```python
from build123d import *

# Parameters (mm, degrees)
SKETCH1_R           = 19.36
BOSS_EXTRUDE1_DEPTH = 10
CUT_EXTRUDE1_REACH  = 12
CUT_EXTRUDE2_REACH  = 12
SKETCH3_R           = 9.21
SKETCH4_R           = 19.36
SKETCH4_R_2         = 9.21
BOSS_EXTRUDE2_DEPTH = 2
SKETCH5_R           = 19.522617412
SKETCH5_R_2         = 17.522617412
BOSS_EXTRUDE3_DEPTH = 12


with BuildPart() as part:
    # Sketch1 → Boss-Extrude1 (new body)
    with BuildSketch(Plane(origin=(0, 0, 0), x_dir=(1, 0, 0), z_dir=(0, 1, 0))):
        Circle(SKETCH1_R)
    extrude(amount=BOSS_EXTRUDE1_DEPTH)

    # Sketch2 → Cut-Extrude1 (cut, up to next)
    with BuildSketch(Plane.XZ, mode=Mode.PRIVATE) as cut_extrude1_sk1:
        with BuildLine():
            Line((13.175859246, 14.184721821), (10.029502225, 10.277095169))
            ThreePointArc((10.029502225, 10.277095169), (12.436124798, 7.18), (13.914976606, 3.54725613))
            Line((13.914976606, 3.54725613), (18.872259065, 4.318267913))
            ThreePointArc((18.872259065, 4.318267913), (16.766251817, 9.68), (13.175859246, 14.184721821))
        make_face()
    cut_extrude1_tool1 = extrude(cut_extrude1_sk1.sketch, amount=-CUT_EXTRUDE1_REACH, mode=Mode.PRIVATE) & part.part
    add(cut_extrude1_tool1.solids().sort_by_distance((14.534106, 0, 8.39127))[0], mode=Mode.SUBTRACT)
    # Sketch2 → Cut-Extrude1 (cut, up to next)
    with BuildSketch(Plane.XZ, mode=Mode.PRIVATE) as cut_extrude1_sk2:
        with BuildLine():
            ThreePointArc((-13.914976606, 3.54725613), (-12.436124798, 7.18), (-10.029502225, 10.277095169))
            Line((-10.029502225, 10.277095169), (-13.175859246, 14.184721821))
            ThreePointArc((-13.175859246, 14.184721821), (-16.766251817, 9.68), (-18.872259065, 4.318267913))
            Line((-18.872259065, 4.318267913), (-13.914976606, 3.54725613))
        make_face()
    cut_extrude1_tool2 = extrude(cut_extrude1_sk2.sketch, amount=-CUT_EXTRUDE1_REACH, mode=Mode.PRIVATE) & part.part
    add(cut_extrude1_tool2.solids().sort_by_distance((-14.534106, 0, 8.39127))[0], mode=Mode.SUBTRACT)
    # Sketch2 → Cut-Extrude1 (cut, up to next)
    with BuildSketch(Plane.XZ, mode=Mode.PRIVATE) as cut_extrude1_sk3:
        with BuildLine():
            Line((5.69639982, -18.502989734), (3.885474381, -13.824351299))
            ThreePointArc((3.885474381, -13.824351299), (0, -14.36), (-3.885474381, -13.824351299))
            Line((-3.885474381, -13.824351299), (-5.69639982, -18.502989734))
            ThreePointArc((-5.69639982, -18.502989734), (0, -19.36), (5.69639982, -18.502989734))
        make_face()
    cut_extrude1_tool3 = extrude(cut_extrude1_sk3.sketch, amount=-CUT_EXTRUDE1_REACH, mode=Mode.PRIVATE) & part.part
    add(cut_extrude1_tool3.solids().sort_by_distance((0, 0, -16.782541))[0], mode=Mode.SUBTRACT)

    # Sketch3 → Cut-Extrude2 (cut, up to next)
    with BuildSketch(Plane.XZ, mode=Mode.PRIVATE) as cut_extrude2_sk1:
        Circle(SKETCH3_R)
    cut_extrude2_tool1 = extrude(cut_extrude2_sk1.sketch, amount=-CUT_EXTRUDE2_REACH, mode=Mode.PRIVATE) & part.part
    add(cut_extrude2_tool1.solids().sort_by_distance((0, 0, 0))[0], mode=Mode.SUBTRACT)

    # Sketch4 → Boss-Extrude2 (add)
    with BuildSketch(Plane.XZ):
        Circle(SKETCH4_R)
        Circle(SKETCH4_R_2, mode=Mode.SUBTRACT)
    extrude(amount=BOSS_EXTRUDE2_DEPTH)

    # Sketch5 → Boss-Extrude3 (add)
    with BuildSketch(Plane.XZ.offset(2)):
        Circle(SKETCH5_R)
        Circle(SKETCH5_R_2, mode=Mode.SUBTRACT)
    extrude(amount=-BOSS_EXTRUDE3_DEPTH)


solid = part.part
```
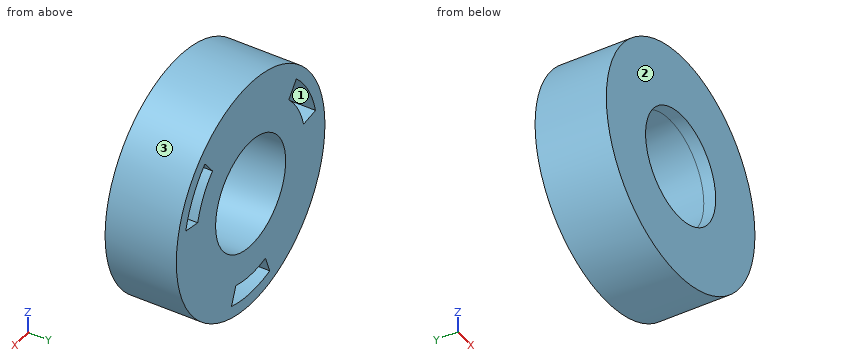
Work out the finished part from the listing and answer in its coordinate system (mm). Face numbers are marked on the shaded views. Coordinates: 2 decimals unless noted, no trailing zeros. Loops run counter-clockwise (first coordinate to the right, second up) from the corner with the lowest first, then second, coordinate; pieces in that order, holes last. Notation, with made-up numbers: (18.25, -29) -> (47.25, -29) arc R23 cw to (47.25, 9) -> close; hole circle Ø7 at (65.5, 61). An arc over 180 degrees is marked (long way). Answer as CSV lines item,"result".
Q1. The part is cut by section D-D on x = 0. Write down the section's boundary in (y, z), and give its area (3 significant figures).
Findings:
outline,"(-2, -19.52) -> (10, -19.52) -> (10, -17.52) -> (0, -17.52) -> (0, -14.36) -> (10, -14.36) -> (10, -9.21) -> (-2, -9.21) -> close; (-2, 9.21) -> (10, 9.21) -> (10, 19.52) -> (-2, 19.52) -> close"
area,"216 mm²"
Q2. Each of these flat-tipped pins is pushed along its axis until it touches: pin 1 (5 mm diameter, centred on x = 13, y = 6, fed in from +Z); pin 2 (3 mm diameter, centred on y = 2, z = -10.5, fed in from -X); pin 3 (4 mm diameter, centred on x = -11.5, y = 7, fed in from -Z). Where does it stop, or does it pass through?
Findings:
pin 1,"stops at z = 16.46"
pin 2,"stops at x = -17.32"
pin 3,"stops at z = -17.06"
Q3. The part is cut by section C-C on y = 9.25. Write down the section's boundary in (x, z).
Findings:
outline,"circle Ø39.05 at (0, 0); hole (-17.05, 4.04) -> (-13.91, 3.55) arc R14.36 cw to (-10.03, 10.28) -> (-12.02, 12.75) arc R17.52 ccw to start; hole circle Ø18.42 at (0, 0); hole (-5.03, -16.78) arc R17.52 ccw to (5.03, -16.78) -> (3.89, -13.82) arc R14.36 cw to (-3.89, -13.82) -> close; hole (10.03, 10.28) arc R14.36 cw to (13.91, 3.55) -> (17.05, 4.04) arc R17.52 ccw to (12.02, 12.75) -> close"
Q4. For a pull along X with two mould halves and no side action, classify the marked faces 1, 2 and 3 as +X half, -X half, draft (parallel to the pull), parting line (faces both ways), or undercut.
Findings:
face 1,"undercut"
face 2,"draft"
face 3,"parting line"
Q5. The part is cut by section B-B on x = 6.5. Write down the section's boundary in (y, z), and give its area (3 significant figures).
Findings:
outline,"(-2, -18.41) -> (10, -18.41) -> (10, -6.52) -> (-2, -6.52) -> close; (-2, 6.52) -> (10, 6.52) -> (10, 18.41) -> (-2, 18.41) -> close"
area,"285 mm²"
Q6. The part is cut by section A-A on z = 0. Write down the section's boundary in (x, y).
Findings:
outline,"(-19.52, -2) -> (-9.21, -2) -> (-9.21, 10) -> (-19.52, 10) -> close; (9.21, -2) -> (19.52, -2) -> (19.52, 10) -> (9.21, 10) -> close"
Q7. Find the intervals of material crossed by probe 1 along Z at (x, y) = (0, 3); probe 2 along X at (y, z) = (4, 11.5); probe 3 along Z at (x, y) = (-2, 6.25), in increasing order.
Findings:
probe 1,"z = -19.52 to -17.52, -14.36 to -9.21, 9.21 to 19.52"
probe 2,"x = -15.78 to -13.22, -11.01 to 11.01, 13.22 to 15.78"
probe 3,"z = -19.42 to -17.41, -14.22 to -8.99, 8.99 to 19.42"
